The listing builds one solid part. Answer for the finished solid, in the listing's coordinates (mm). A direction names the side the tool comes from. Coordinates: 2 decimals unless noted, no trailing zeros. Order: outer loops, then holes, each group sorted by start corner. A loop starts at its lowest first (then second) coordinate and runs counter-clockwise, first axis right, second up. Notation, with made-up numbers: (-40, 33) -> (-16, 33) arc R36 cw to (-16, 72) -> close; hole circle Ø2 at (42.5, 17). An arc over 180 degrees is marked (long way). Return JSON: item names as keys, results as strings.
```python
from build123d import *

# Parameters (mm, degrees)
SKETCH1_R                    = 3.25
BASE_FLANGE1_DEPTH           = 3.175
EDGE_FLANGE1_STRIP_W         = 14.1732
EDGE_FLANGE1_STRIP_H         = 3.175
EDGE_FLANGE1_STRIP_CUT_DEPTH = 14
EDGE_FLANGE1_DEPTH           = 14
EDGE_FLANGE2_STRIP_W         = 14.1732
EDGE_FLANGE2_STRIP_H         = 3.175
EDGE_FLANGE2_STRIP_CUT_DEPTH = 14
EDGE_FLANGE2_DEPTH           = 14
SKETCH17_R                   = 3.175
CUT_EXTRUDE1_DEPTH           = 3.175


# Sheet-metal steps are written as plain solids
with BuildPart() as part:
    # Sketch1 → Base-Flange1 (new body)
    with BuildSketch(Plane(origin=(0, 0, 0), x_dir=(1, 0, 0), z_dir=(0, 1, 0))):
        with BuildLine():
            Line((12.950003607, 12.5), (-1.049996393, 12.5))
            Line((-1.049996393, 12.5), (-1.049996393, 9.5))
            ThreePointArc((-1.049996393, 9.5), (-1.120300603, 9.131671699), (-1.321327868, 8.815133458))
            Line((-1.321327868, 8.815133458), (-5.100679674, 4.794065797))
            ThreePointArc((-5.100679674, 4.794065797), (-6.725789914, 0.499030469), (-4.837867779, -3.687144607))
            Line((-4.837867779, -3.687144607), (-3.380530729, -5.056877692))
            ThreePointArc((-3.380530729, -5.056877692), (0.914504598, -6.681987931), (5.100679674, -4.794065797))
            Line((5.100679674, -4.794065797), (8.88003148, -0.772998135))
            ThreePointArc((8.88003148, -0.772998135), (11.895440461, 3.97507548), (12.950003607, 9.5))
            Line((12.950003607, 9.5), (12.950003607, 12.5))
        make_face()
        with Locations(Location((0, 0, 0), (0, 0, 270))):
            Circle(SKETCH1_R, mode=Mode.SUBTRACT)
    extrude(amount=-BASE_FLANGE1_DEPTH)

    # Edge-Flange1 strip (across the edge) → Edge-Flange1 strip cut (cut)
    with BuildSketch(Plane(origin=(12.950003607, 0, -12.5), x_dir=(0, 0, 1), z_dir=(-1, 0, 0))):
        with Locations((-6.35, -1.5875)):
            Rectangle(EDGE_FLANGE1_STRIP_W, EDGE_FLANGE1_STRIP_H)
    extrude(amount=EDGE_FLANGE1_STRIP_CUT_DEPTH, mode=Mode.SUBTRACT)

    # Edge-Flange1 section (across the edge) → Edge-Flange1 (add)
    with BuildSketch(Plane(origin=(12.950003607, 0, -12.5), x_dir=(0, 0, 1), z_dir=(-1, 0, 0))):
        with BuildLine():
            Line((-3.175, 0.7366), (-3.175, 7.324994814))
            Line((-3.175, 7.324994814), (0, 7.324994814))
            Line((0, 7.324994814), (0, 0.7366))
            ThreePointArc((0, 0.7366), (0.215745145, 0.215745145), (0.7366, 0))
            Line((0.7366, 0), (0.7366, -3.175))
            ThreePointArc((0.7366, -3.175), (-2.029318885, -2.029318885), (-3.175, 0.7366))
        make_face()
    extrude(amount=EDGE_FLANGE1_DEPTH)

    # Edge-Flange2 strip (across the edge) → Edge-Flange2 strip cut (cut)
    with BuildSketch(Plane(origin=(-1.049996393, 7.324994814, -15.675), x_dir=(0, -1, 0), z_dir=(1, 0, 0))):
        with Locations((-3.175, -1.5875)):
            Rectangle(EDGE_FLANGE2_STRIP_W, EDGE_FLANGE2_STRIP_H)
    extrude(amount=EDGE_FLANGE2_STRIP_CUT_DEPTH, mode=Mode.SUBTRACT)

    # Edge-Flange2 section (across the edge) → Edge-Flange2 (add)
    with BuildSketch(Plane(origin=(-1.049996393, 7.324994814, -15.675), x_dir=(0, -1, 0), z_dir=(1, 0, 0))):
        with BuildLine():
            Line((0, 0.7366), (0, 40.174998631))
            Line((0, 40.174998631), (3.175, 40.174998631))
            Line((3.175, 40.174998631), (3.175, 0.7366))
            ThreePointArc((3.175, 0.7366), (3.390745145, 0.215745145), (3.9116, 0))
            Line((3.9116, 0), (3.9116, -3.175))
            ThreePointArc((3.9116, -3.175), (1.145681115, -2.029318885), (0, 0.7366))
        make_face()
    extrude(amount=EDGE_FLANGE2_DEPTH)

    # Sketch17 → Cut-Extrude1 (cut)
    with BuildSketch(Plane(origin=(0, 7.324994814, 0), x_dir=(1, 0, 0), z_dir=(0, 1, 0))):
        with BuildLine():
            ThreePointArc((-1.049996393, 48.849998631), (1.000256139, 53.7997461), (5.950003607, 55.849998631))
            Line((5.950003607, 55.849998631), (-1.049996393, 55.849998631))
            Line((-1.049996393, 55.849998631), (-1.049996393, 48.849998631))
        make_face()
        with BuildLine():
            ThreePointArc((5.950003607, 55.849998631), (10.899751075, 53.7997461), (12.950003607, 48.849998631))
            Line((12.950003607, 48.849998631), (12.950003607, 55.849998631))
            Line((12.950003607, 55.849998631), (5.950003607, 55.849998631))
        make_face()
        with Locations(Location((5.950003607, 48.849998631, 0), (0, 0, 270))):
            Circle(SKETCH17_R)
    extrude(amount=-CUT_EXTRUDE1_DEPTH, mode=Mode.SUBTRACT)


solid = part.part
```
Item 1: The part is cut by section A-A on z = 0. Determine the outline of the cut face in (x, y) (3 decimals), plus the area to 3 significant figures.
Answer list:
{"outline": "(-6.689, -3.175) -> (-3.25, -3.175) -> (-3.25, 0) -> (-6.689, 0) -> close; (3.25, -3.175) -> (9.558, -3.175) -> (9.558, 0) -> (3.25, 0) -> close", "area": "30.9 mm2"}
Item 2: Which of the six approach directions +Z, -Z, +X, -X, +Y, -Y give full straight-line access (tool end or side, diameter ignored) to faces 1 (the flat face through (6, 2, -15.675)), 2 (the flat face through (-1.05, 4.4, -27.8)), 3 (the flat face through (3, 0, -3))?
Answer list:
{"face 1": "-Z, +X, -X, -Y", "face 2": "-Z, -X, +Y, -Y", "face 3": "+Z, +X, -X, +Y"}
Item 3: The part is cut by section C-C on y = 6.75. Determine the outline of the cut face in (x, z) (3 decimals).
Answer list:
{"outline": "(-1.05, -48.85) arc R7 ccw to (12.95, -48.85) -> (12.95, -14.37) -> (-1.05, -14.37) -> close; hole circle Ø6.35 at (5.95, -48.85)"}
Item 4: Find the intervals of material crossed by probe 1 along X at (y, z) = (-1, 0); probe 2 along Y at (x, z) = (9.25, -48) (3 decimals); probe 3 along Z at (x, y) = (4.25, 1) (3 decimals), in increasing order.
Answer list:
{"probe 1": "-6.69 to -3.25, 3.25 to 9.56", "probe 2": "4.15 to 7.325", "probe 3": "-15.675 to -12.5"}
Item 5: Determine the mould class of faces 4 (the cylindrical face through (-1.978, -1.565, -2.579)), 5 (the flat face through (-4.12, -1.57, 4.36)), 6 (the flat face through (6.964, -1.565, 2.812)), 7 (the flat face through (3, -3.175, -3)) for opening direction X: pulls with the +X half, pulls with the -X half, needs draft (parallel to the pull), parting line crosses it, or undercut.
Answer list:
{"face 4": "undercut", "face 5": "pulls with the -X half", "face 6": "pulls with the +X half", "face 7": "needs draft"}
Item 6: The part is cut by section B-B on x = 0. Determine the outline of the cut face in (y, z) (3 decimals), plus the area to 3 significant figures.
Answer list:
{"outline": "(-3.175, -11.763) arc R3.912 ccw to (0.737, -15.675) -> (3.413, -15.675) arc R0.737 cw to (4.15, -16.412) -> (4.15, -52.537) -> (7.325, -52.537) -> (7.325, -16.412) arc R3.912 ccw to (3.413, -12.5) -> (0.737, -12.5) arc R0.737 cw to (0, -11.763) -> (0, -3.25) -> (-3.175, -3.25) -> close; (-3.175, 3.25) -> (0, 3.25) -> (0, 6.64) -> (-3.175, 6.64) -> close", "area": "184 mm2"}
Item 7: Flat-ended cylindrical pins translate along their axes: pin 1 (3 mm diameter, centred on x = 4.5, y = 3.5, fed in from +Z); pin 2 (5.5 mm diameter, centred on x = 7.5, z = -6.5, fed in from +Y); pin 3 (1.3 mm diameter, centred on x = 8, y = 1.5, fed in from -Z) (3 decimals). Find the tip coordinate at first contact, or state that the pin passes through.
Answer list:
{"pin 1": "z = -12.5", "pin 2": "y = 0", "pin 3": "z = -15.675"}
Item 8: The part is cut by section D-D on x = 11. Determine the outline of the cut face in (y, z) (3 decimals), plus the area to 3 significant figures.
Answer list:
{"outline": "(-3.175, -11.763) arc R3.912 ccw to (0.737, -15.675) -> (3.413, -15.675) arc R0.737 cw to (4.15, -16.412) -> (4.15, -53.697) -> (7.325, -53.697) -> (7.325, -16.412) arc R3.912 ccw to (3.413, -12.5) -> (0.737, -12.5) arc R0.737 cw to (0, -11.763) -> (0, -2.104) -> (-3.175, -2.104) -> close", "area": "181 mm2"}
